```python
from build123d import *

# Parameters (mm, degrees)
SKETCH1_W             = 42
SKETCH1_H             = 10
BOSS_EXTRUDE1_DEPTH   = 3
F_5_0MM_DOWEL_HOLE1_D = 5
F_3_0MM_DOWEL_HOLE1_D = 3
SKETCH2_R             = 1
CUT_EXTRUDE1_DEPTH    = 3
FILLET1_R             = 3


with BuildPart() as part:
    # Sketch1 → Boss-Extrude1 (new body)
    with BuildSketch(Plane(origin=(0, 0, 0), x_dir=(1, 0, 0), z_dir=(0, 1, 0))):
        Rectangle(SKETCH1_W, SKETCH1_H)
    extrude(amount=BOSS_EXTRUDE1_DEPTH)

    # Ø5.0mm Dowel Hole1 (through all)
    with Locations(Plane(origin=(0, 3, 0), x_dir=(1, 0, 0), z_dir=(0, 1, 0))):
        with Locations((15, 0)):
            Hole(F_5_0MM_DOWEL_HOLE1_D / 2)

    # Ø3.0mm Dowel Hole1 (through all)
    with Locations(Plane(origin=(0, 3, 0), x_dir=(1, 0, 0), z_dir=(0, 1, 0))):
        with Locations((-15, 0)):
            Hole(F_3_0MM_DOWEL_HOLE1_D / 2)

    # Sketch2 → Cut-Extrude1 (cut)
    with BuildSketch(Plane(origin=(0, 3, 0), x_dir=(1, 0, 0), z_dir=(0, 1, 0))):
        with Locations((6.55, 0)):
            Circle(SKETCH2_R)
        with Locations((2.55, 0)):
            Circle(SKETCH2_R)
    extrude(amount=-CUT_EXTRUDE1_DEPTH, mode=Mode.SUBTRACT)

    # Fillet1
    fillet1_edges = [part.edges().sort_by_distance(p)[0] for p in [
        (21, 1.5, 5),
        (-21, 1.5, 5),
        (-21, 1.5, -5),
        (21, 1.5, -5),
    ]]
    fillet(fillet1_edges, radius=FILLET1_R)


solid = part.part
```
Part model, mm, in its own coordinate system. Coordinates: 2 decimals unless noted, no trailing zeros. Write each loop counter-clockwise with the first axis right and the second up, starting at its lowest first coordinate (ties: lowest second). Pieces come first, ordered by that corner, then holes.
Item 1: Slice it at C-C (x = 15). Write the cut outline in (y, z).
Item 2: Slice it at A-A (y = 2.55). Write the cut outline in (x, z).
Item 3: Slice it at D-D (z = 4.5). Write the cut outline in (x, y), and give its area (3 significant figures).
Item 4: Probe line 1 (Z direction, x = 6.55, y = 2.3); line 2 (X direction, y = 1.4, z = -0.5); line 3 (Z direction, x = -15, y = 2.45). List the from-to ranges inside material, lowest first.
Item 5: Slice it at B-B (x = 2.55). Write the cut outline in (y, z).
Item 6: Pin check, flat tip, straight feed: pin 1 (5 mm diameter, centred on x = 1, z = -2.5, fed in from -Y). Stop position of the tip, or through.
Item 7: Mould opens along X. For faces 1 (the face through (5.55, 1.52, -0.04)), 2 (the face through (0, 1, 5)), 3 (the face through (20.1, 1.52, -4.14)) say: released by +X, released by -X, zero draft, split by the parting line, or undercut.
Results found:
1. outline: (0, -5) - (3, -5) - (3, -2.5) - (0, -2.5) - close; (0, 2.5) - (3, 2.5) - (3, 5) - (0, 5) - close
2. outline: (-21, -2) arc R3 ccw to (-18, -5) - (18, -5) arc R3 ccw to (21, -2) - (21, 2) arc R3 ccw to (18, 5) - (-18, 5) arc R3 ccw to (-21, 2) - close; hole circle Ø3 at (-15, 0); hole circle Ø2 at (2.55, 0); hole circle Ø2 at (6.55, 0); hole circle Ø5 at (15, 0)
3. outline: (-19.66, 0) - (19.66, 0) - (19.66, 3) - (-19.66, 3) - close
3. area: 118 mm2
4. line 1: z = -5 to -1, 1 to 5
4. line 2: x = -21 to -16.41, -13.59 to 1.68, 3.42 to 5.68, 7.42 to 12.55, 17.45 to 21
4. line 3: z = -5 to -1.5, 1.5 to 5
5. outline: (0, -5) - (3, -5) - (3, -1) - (0, -1) - close; (0, 1) - (3, 1) - (3, 5) - (0, 5) - close
6. pin 1: stops at y = 0
7. face 1: undercut
7. face 2: zero draft
7. face 3: released by +X
